Geometry: final body of the model. Coordinates: model frame, mm. Give positions to 0.01 mm unless a question says otherwise; leave off trailing zeros. Write each loop counter-clockwise with the first axis right and the second up, starting at its lowest first coordinate (ties: lowest second). Pieces come first, ordered by that corner, then holes. Notation, with made-up numbers: M 80,51.5 L 122,51.5 A24 ccw 122,79.5 Z; hole C 18,57.25 d4. An arc over 180 degrees is marked long. Use a Markdown table: item, result. Add a question column.
(1) Pin query (flat end, axial travel): pin 1 Ø1.8 at (x, z) = (53.98, 105) entering from -Y; pin 2 Ø2.5 at (y, z) = (3.5, -129.5) entering from +X; pin 3 Ø2.5 at (x, y) = (73.5, 1.5) entering from +Z; pin 4 Ø2 at (x, y) = (-78, 2) entering from -Z. Return the tip coordinate at first contact, or that it passes through.
(2) Cut plane D-D (y = 2.3). State how many separate pieces and enclosed holes the cut face has, plus the area to 3 significant figures.
(3) Cut plane A-A (x = 65). Output: boundary loops of the cut face in (y, z), plus the area to 3 significant figures.
(4) Cut plane C-C (z = -39.5). Output: boundary loops of the cut face in (x, y), plus the area to 3 significant figures.
(5) Cut plane B-B (x = -24). Output: boundary loops of the cut face in (y, z).
(6) Material intervals for L1, parallel to Z at x = -10, y = 0.5; L2, parallel to Z at x = 54, y = 0.85; L3, parallel to X at y = 1.6, z = -105, sorted ascending.
```python
from build123d import *

# Parameters (mm, degrees)
ESQUISSE1_R        = 1.5
ESQUISSE1_W        = 97.855109658
ESQUISSE1_H        = 40
BOSS_EXTRU_1_DEPTH = 5


with BuildPart() as part:
    # Esquisse1 → Boss.-Extru.1 (new body)
    with BuildSketch(Plane(origin=(0, 0, 0), x_dir=(1, 0, 0), z_dir=(0, 1, 0))):
        Polygon((-58.927554829, 110), (-58.927554829, 160), (58.927554829, 160), (58.927554829, 110), (108.927554829, 110), (108.927554829, -110), (58.927554829, -110), (58.927554829, -160), (-58.927554829, -160), (-58.927554829, -110), (-108.927554829, -110), (-108.927554829, -50), (98.927554829, -50), (98.927554829, 50), (-108.927554829, 50), (-108.927554829, 110), align=None)
        with Locations(Location((-103.976302336, -105, 0), (0, 0, 270))):
            Circle(ESQUISSE1_R, mode=Mode.SUBTRACT)
        with Locations(Location((-103.976302336, -55, 0), (0, 0, 270))):
            Circle(ESQUISSE1_R, mode=Mode.SUBTRACT)
        with Locations(Location((-53.976302336, -105, 0), (0, 0, 270))):
            Circle(ESQUISSE1_R, mode=Mode.SUBTRACT)
        with Locations(Location((-53.976302336, -155, 0), (0, 0, 270))):
            Circle(ESQUISSE1_R, mode=Mode.SUBTRACT)
        with Locations(Location((-53.976302336, 155, 0), (0, 0, 90))):
            Circle(ESQUISSE1_R, mode=Mode.SUBTRACT)
        with Locations(Location((-53.976302336, 105, 0), (0, 0, 90))):
            Circle(ESQUISSE1_R, mode=Mode.SUBTRACT)
        with Locations(Location((-103.976302336, 105, 0), (0, 0, 90))):
            Circle(ESQUISSE1_R, mode=Mode.SUBTRACT)
        with Locations(Location((-103.976302336, 55, 0), (0, 0, 90))):
            Circle(ESQUISSE1_R, mode=Mode.SUBTRACT)
        with Locations(Location((53.976302336, -155, 0), (0, 0, 90))):
            Circle(ESQUISSE1_R, mode=Mode.SUBTRACT)
        with Locations(Location((53.976302336, -105, 0), (0, 0, 90))):
            Circle(ESQUISSE1_R, mode=Mode.SUBTRACT)
        with Locations(Location((103.976302336, -105, 0), (0, 0, 90))):
            Circle(ESQUISSE1_R, mode=Mode.SUBTRACT)
        with Locations(Location((103.976302336, 105, 0), (0, 0, 270))):
            Circle(ESQUISSE1_R, mode=Mode.SUBTRACT)
        with Locations(Location((53.976302336, 105, 0), (0, 0, 270))):
            Circle(ESQUISSE1_R, mode=Mode.SUBTRACT)
        with Locations(Location((53.976302336, 155, 0), (0, 0, 270))):
            Circle(ESQUISSE1_R, mode=Mode.SUBTRACT)
        with Locations((0, -130)):
            Rectangle(ESQUISSE1_W, ESQUISSE1_H, mode=Mode.SUBTRACT)
        with Locations((0, 130)):
            Rectangle(ESQUISSE1_W, ESQUISSE1_H, mode=Mode.SUBTRACT)
    extrude(amount=BOSS_EXTRU_1_DEPTH)


solid = part.part
```
Answer list:
| question | item | result |
|---|---|---|
| 1 | pin 1 | through |
| 1 | pin 2 | x = 58.93 |
| 1 | pin 3 | z = 110 |
| 1 | pin 4 | z = -110 |
| 2 | separate pieces | 1 |
| 2 | enclosed holes | 16 |
| 2 | area | 31,000 mm² |
| 3 | outline | M 0,-110 L 5,-110 L 5,-50 L 0,-50 Z; M 0,50 L 5,50 L 5,110 L 0,110 Z |
| 3 | area | 600 mm² |
| 4 | outline | M 98.93,0 L 108.93,0 L 108.93,5 L 98.93,5 Z |
| 4 | area | 50.0 mm² |
| 5 | outline | M 0,-160 L 5,-160 L 5,-150 L 0,-150 Z; M 0,-110 L 5,-110 L 5,-50 L 0,-50 Z; M 0,50 L 5,50 L 5,110 L 0,110 Z; M 0,150 L 5,150 L 5,160 L 0,160 Z |
| 6 | L1 | -160 to -150, -110 to -50, 50 to 110, 150 to 160 |
| 6 | L2 | -160 to -156.5, -153.5 to -106.5, -103.5 to -50, 50 to 103.5, 106.5 to 153.5, 156.5 to 160 |
| 6 | L3 | -108.93 to -105.48, -102.48 to -55.48, -52.48 to 52.48, 55.48 to 102.48, 105.48 to 108.93 |
